Here's how the part is built. I have some questions about the finished solid (model axes, mm). A direction names the side the tool comes from. Round coordinates to 2 decimals unless told otherwise and drop trailing zeros. Order: outer loops, then holes, each group sorted by start corner. A loop starts at its lowest first (then second) coordinate and runs counter-clockwise, first axis right, second up. Notation, with made-up numbers: (36.5, 62.5) - (53.5, 62.5) arc R29 cw to (53.5, 99.5) - close; hole circle Ø1 at (-32, -29). An arc over 180 degrees is marked (long way). Answer as a JSON object with one key per item and string values.
```python
from build123d import *

# Parameters (mm, degrees)
CYLINDER324_R     = 2
CYLINDER324_DEPTH = 47
CYLINDER323_R     = 2
CYLINDER323_DEPTH = 47
BOX411_W          = 6
BOX411_H          = 15
BOX411_DEPTH      = 25
BOX409_W          = 6
BOX409_H          = 15
BOX409_DEPTH      = 25
BOX410_W          = 16
BOX410_H          = 15
BOX410_DEPTH      = 5
BOX412_W          = 16
BOX412_H          = 15
BOX412_DEPTH      = 5
BOX430_W          = 6
BOX430_H          = 9
BOX430_DEPTH      = 20.1
CYLINDER180_R     = 2
CYLINDER180_DEPTH = 33
CYLINDER179_R     = 2
CYLINDER179_DEPTH = 30
CYLINDER182_R     = 2
CYLINDER182_DEPTH = 33
CYLINDER181_R     = 2
CYLINDER181_DEPTH = 30
BOX281_W          = 27.3
BOX281_H          = 9
BOX281_DEPTH      = 20.1
BOX408_W          = 27.3
BOX408_H          = 9
BOX408_DEPTH      = 20.1
BOX283_W          = 66
BOX283_H          = 58.1
BOX283_DEPTH      = 3
CYLINDER326_R     = 2
CYLINDER326_DEPTH = 47
CYLINDER325_R     = 2
CYLINDER325_DEPTH = 47
BOX286_W          = 6
BOX286_H          = 20
BOX286_DEPTH      = 25
BOX407_W          = 16
BOX407_H          = 20
BOX407_DEPTH      = 5
BOX288_W          = 6
BOX288_H          = 20
BOX288_DEPTH      = 25
BOX406_W          = 16
BOX406_H          = 20
BOX406_DEPTH      = 5


with BuildPart() as cylinder324:
    # Cylinder324 → Cylinder324 (new body)
    with BuildSketch(Plane(origin=(-75, -98, -5), x_dir=(1, 0, 0), z_dir=(0, 0, 1))):
        Circle(CYLINDER324_R)
    extrude(amount=CYLINDER324_DEPTH)


with BuildPart() as fusion314:
    # Cylinder323 → Cylinder323 (new body)
    with BuildSketch(Plane(origin=(7, -98, -5), x_dir=(1, 0, 0), z_dir=(0, 0, 1))):
        Circle(CYLINDER323_R)
    extrude(amount=CYLINDER323_DEPTH)

    # Fusion314: union Cylinder324
    add(cylinder324.part)


with BuildPart() as fusion314_1:
    # Fusion314 placement: moved
    add(fusion314.part.moved(Location((0, 41, 0))))


with BuildPart() as box411:
    # Box411 → Box411 (new body)
    with BuildSketch(Plane(origin=(-6.9, -64.9, 37), x_dir=(1, 0, 0), z_dir=(0, 0, 1))):
        with Locations((3, 7.5)):
            Rectangle(BOX411_W, BOX411_H)
    extrude(amount=BOX411_DEPTH)


with BuildPart() as box409:
    # Box409 → Box409 (new body)
    with BuildSketch(Plane(origin=(-66.9, -64.9, 37), x_dir=(1, 0, 0), z_dir=(0, 0, 1))):
        with Locations((3, 7.5)):
            Rectangle(BOX409_W, BOX409_H)
    extrude(amount=BOX409_DEPTH)


with BuildPart() as box410:
    # Box410 → Box410 (new body)
    with BuildSketch(Plane(origin=(-82.9, -64.9, 37), x_dir=(1, 0, 0), z_dir=(0, 0, 1))):
        with Locations((8, 7.5)):
            Rectangle(BOX410_W, BOX410_H)
    extrude(amount=BOX410_DEPTH)


with BuildPart() as cut338:
    # Box412 → Box412 (new body)
    with BuildSketch(Plane(origin=(-0.9, -64.9, 37), x_dir=(1, 0, 0), z_dir=(0, 0, 1))):
        with Locations((8, 7.5)):
            Rectangle(BOX412_W, BOX412_H)
    extrude(amount=BOX412_DEPTH)

    # Fusion322: union Box411, Box409, Box410
    add(box411.part)
    add(box409.part)
    add(box410.part)

    # Cut338: cut Fusion314
    add(fusion314_1.part, mode=Mode.SUBTRACT)


with BuildPart() as box430:
    # Box430 → Box430 (new body)
    with BuildSketch(Plane(origin=(-66.5, -108, 62), x_dir=(1, 0, 0), z_dir=(0, 0, 1))):
        with Locations((3, 4.5)):
            Rectangle(BOX430_W, BOX430_H)
    extrude(amount=BOX430_DEPTH)


with BuildPart() as cylinder180:
    # Cylinder180 → Cylinder180 (new body)
    with BuildSketch(Plane(origin=(-74.6, -105.8, 63), x_dir=(0, 0, -1), z_dir=(1, 0, 0))):
        Circle(CYLINDER180_R)
    extrude(amount=CYLINDER180_DEPTH)


with BuildPart() as fusion247:
    # Cylinder179 → Cylinder179 (new body)
    with BuildSketch(Plane(origin=(-71.6, -105.8, 73), x_dir=(0, 0, -1), z_dir=(1, 0, 0))):
        Circle(CYLINDER179_R)
    extrude(amount=CYLINDER179_DEPTH)

    # Fusion247: union Cylinder180
    add(cylinder180.part)


with BuildPart() as fusion247_1:
    # Fusion247 placement: moved
    add(fusion247.part.moved(Location((0, 2, 4))))


with BuildPart() as cylinder182:
    # Cylinder182 → Cylinder182 (new body)
    with BuildSketch(Plane(origin=(-74.6, -56.2, 63), x_dir=(0, 0, -1), z_dir=(1, 0, 0))):
        Circle(CYLINDER182_R)
    extrude(amount=CYLINDER182_DEPTH)


with BuildPart() as fusion252:
    # Cylinder181 → Cylinder181 (new body)
    with BuildSketch(Plane(origin=(-71.6, -56.2, 73), x_dir=(0, 0, -1), z_dir=(1, 0, 0))):
        Circle(CYLINDER181_R)
    extrude(amount=CYLINDER181_DEPTH)

    # Fusion246: union Cylinder182
    add(cylinder182.part)


with BuildPart() as fusion252_1:
    # Fusion246 placement: moved
    add(fusion252.part.moved(Location((0, 2, 4))))

    # Fusion252: union Fusion247
    add(fusion247_1.part)


with BuildPart() as box281:
    # Box281 → Box281 (new body)
    with BuildSketch(Plane(origin=(-71.6, -108, 62), x_dir=(1, 0, 0), z_dir=(0, 0, 1))):
        with Locations((13.65, 4.5)):
            Rectangle(BOX281_W, BOX281_H)
    extrude(amount=BOX281_DEPTH)


with BuildPart() as box408:
    # Box408 → Box408 (new body)
    with BuildSketch(Plane(origin=(-71.6, -58.9, 62), x_dir=(1, 0, 0), z_dir=(0, 0, 1))):
        with Locations((13.65, 4.5)):
            Rectangle(BOX408_W, BOX408_H)
    extrude(amount=BOX408_DEPTH)


with BuildPart() as cut336:
    # Box283 → Box283 (new body)
    with BuildSketch(Plane(origin=(-71.6, -108, 59), x_dir=(1, 0, 0), z_dir=(0, 0, 1))):
        with Locations((33, 29.05)):
            Rectangle(BOX283_W, BOX283_H)
    extrude(amount=BOX283_DEPTH)

    # Fusion251: union Box281, Box408
    add(box281.part)
    add(box408.part)

    # Cut283: cut Fusion252
    add(fusion252_1.part, mode=Mode.SUBTRACT)

    # Cut336: cut Box430
    add(box430.part, mode=Mode.SUBTRACT)


with BuildPart() as cut336_1:
    # Cut336 placement: moved
    add(cut336.part.moved(Location((4.7, 0, 0))))


with BuildPart() as cylinder326:
    # Cylinder326 → Cylinder326 (new body)
    with BuildSketch(Plane(origin=(-75, -98, -5), x_dir=(1, 0, 0), z_dir=(0, 0, 1))):
        Circle(CYLINDER326_R)
    extrude(amount=CYLINDER326_DEPTH)


with BuildPart() as fusion315:
    # Cylinder325 → Cylinder325 (new body)
    with BuildSketch(Plane(origin=(7, -98, -5), x_dir=(1, 0, 0), z_dir=(0, 0, 1))):
        Circle(CYLINDER325_R)
    extrude(amount=CYLINDER325_DEPTH)

    # Fusion315: union Cylinder326
    add(cylinder326.part)


with BuildPart() as box286:
    # Box286 → Box286 (new body)
    with BuildSketch(Plane(origin=(-66.9, -108, 37), x_dir=(1, 0, 0), z_dir=(0, 0, 1))):
        with Locations((3, 10)):
            Rectangle(BOX286_W, BOX286_H)
    extrude(amount=BOX286_DEPTH)


with BuildPart() as box407:
    # Box407 → Box407 (new body)
    with BuildSketch(Plane(origin=(-0.9, -108, 37), x_dir=(1, 0, 0), z_dir=(0, 0, 1))):
        with Locations((8, 10)):
            Rectangle(BOX407_W, BOX407_H)
    extrude(amount=BOX407_DEPTH)


with BuildPart() as box288:
    # Box288 → Box288 (new body)
    with BuildSketch(Plane(origin=(-6.9, -108, 37), x_dir=(1, 0, 0), z_dir=(0, 0, 1))):
        with Locations((3, 10)):
            Rectangle(BOX288_W, BOX288_H)
    extrude(amount=BOX288_DEPTH)


with BuildPart() as fusion324:
    # Box406 → Box406 (new body)
    with BuildSketch(Plane(origin=(-82.9, -108, 37), x_dir=(1, 0, 0), z_dir=(0, 0, 1))):
        with Locations((8, 10)):
            Rectangle(BOX406_W, BOX406_H)
    extrude(amount=BOX406_DEPTH)

    # Fusion249: union Box286, Box407, Box288
    add(box286.part)
    add(box407.part)
    add(box288.part)

    # Cut337: cut Fusion315
    add(fusion315.part, mode=Mode.SUBTRACT)

    # Fusion324: union Cut338, Cut336
    add(cut338.part)
    add(cut336_1.part)


solid = fusion324.part
```
1. Imagine slicing it at B-B (y = -103.8). Give the number of separate pieces and of enclosed holes in the cut face, plus the area to 3 significant figures.
Responses:
{"separate pieces": "5", "enclosed holes": "0", "area": "880 mm2"}
2. If I drill on L1, parallel to Y at x = -51.75, z = 67; L2, parallel to Z at x = -65.2, y = -103.8; L3, parallel to Y at x = 7, z = 38.65, over which ranges is the centre line in solid material (lowest first)? Write a range as [from, to].
Responses:
{"L1": "[-108, -105.8], [-101.8, -99], [-58.9, -56.2], [-52.2, -49.9]", "L2": "[37, 65], [69, 75], [79, 82.1]", "L3": "[-108, -100], [-96, -88], [-64.9, -59], [-55, -49.9]"}
3. Imagine slicing it at C-C (x = -59.5). List the corners of the cut face in (y, z) for me, plus the area to 3 significant figures.
Responses:
{"outline": "(-108, 59) - (-49.9, 59) - (-49.9, 82.1) - (-58.9, 82.1) - (-58.9, 62) - (-108, 62) - close; hole circle Ø4 at (-54.2, 67); hole circle Ø4 at (-54.2, 77)", "area": "330 mm2"}
4. Imagine slicing it at A-A (z = 41). List the corners of the cut face in (x, y) for me, plus the area to 3 significant figures.
Responses:
{"outline": "(-82.9, -108) - (-60.9, -108) - (-60.9, -88) - (-82.9, -88) - close; (-82.9, -64.9) - (-60.9, -64.9) - (-60.9, -49.9) - (-82.9, -49.9) - close; (-6.9, -108) - (15.1, -108) - (15.1, -88) - (-6.9, -88) - close; (-6.9, -64.9) - (15.1, -64.9) - (15.1, -49.9) - (-6.9, -49.9) - close; hole circle Ø4 at (-75, -98); hole circle Ø4 at (-75, -57); hole circle Ø4 at (7, -98); hole circle Ø4 at (7, -57)", "area": "1,490 mm2"}
5. Imagine slicing it at D-D (z = 46.5). List the corners of the cut face in (x, y) for me, plus the area to 3 significant figures.
Responses:
{"outline": "(-66.9, -108) - (-60.9, -108) - (-60.9, -88) - (-66.9, -88) - close; (-66.9, -64.9) - (-60.9, -64.9) - (-60.9, -49.9) - (-66.9, -49.9) - close; (-6.9, -108) - (-0.9, -108) - (-0.9, -88) - (-6.9, -88) - close; (-6.9, -64.9) - (-0.9, -64.9) - (-0.9, -49.9) - (-6.9, -49.9) - close", "area": "420 mm2"}
6. For faces 1 (the face through (-64, -99, 72)), 2 (the face through (-39.6, -54, 72)), 3 (the face through (-55.8, -104, 72)), 4 (the face through (-6.9, -58, 48)), which set-ups out of +Z, -Z, +X, -X, +Y, -Y let a thin tool reach every point of the face, with its end or its side?
Responses:
{"face 1": "+Z, +X, -X", "face 2": "+Z, +X, +Y, -Y", "face 3": "+Z, -Y", "face 4": "-Z, +Y, -Y"}
7. For P1, Ø1, axis at x = -31, y = -70, coming from the -Z side; P2, Ø4, axis at x = -50.5, y = -96, coming from the +Z side; P3, Ø12, axis at y = -91.5, z = 56, coming from the -X side, each with a flat end and sliding along its axis, tell me the tip position at first contact or that it passes through.
Responses:
{"P1": "z = 59", "P2": "z = 62", "P3": "x = -66.9"}
8. Thinking about a two-plate mould opening in X: for faces 5 (the face through (-72, -57, 37)), 6 (the face through (-39.6, -104, 72)), 7 (the face through (-6.9, -98, 48)), 8 (the face through (-82.9, -98, 39)), which applies, pulls with the +X half, pulls with the -X half, needs draft (parallel to the pull), parting line crosses it, or undercut?
Responses:
{"face 5": "needs draft", "face 6": "pulls with the +X half", "face 7": "undercut", "face 8": "pulls with the -X half"}
